Verification items for this drawing (mm, ordinates from the low corner). Round coordinates to 2 decimals unless told otherwise and drop trailing zeros. Loops run counter-clockwise (first coordinate to the right, second up) from the corner with the lowest first, then second, coordinate; pieces in that order, holes last. Notation, with made-up numbers: M -28,88 L -22,88 A29 cw -22,125 Z; hole C 21.5,54.5 d1. An arc over 180 degrees is marked long. Answer in a Markdown table with one row per item. Add a question column.
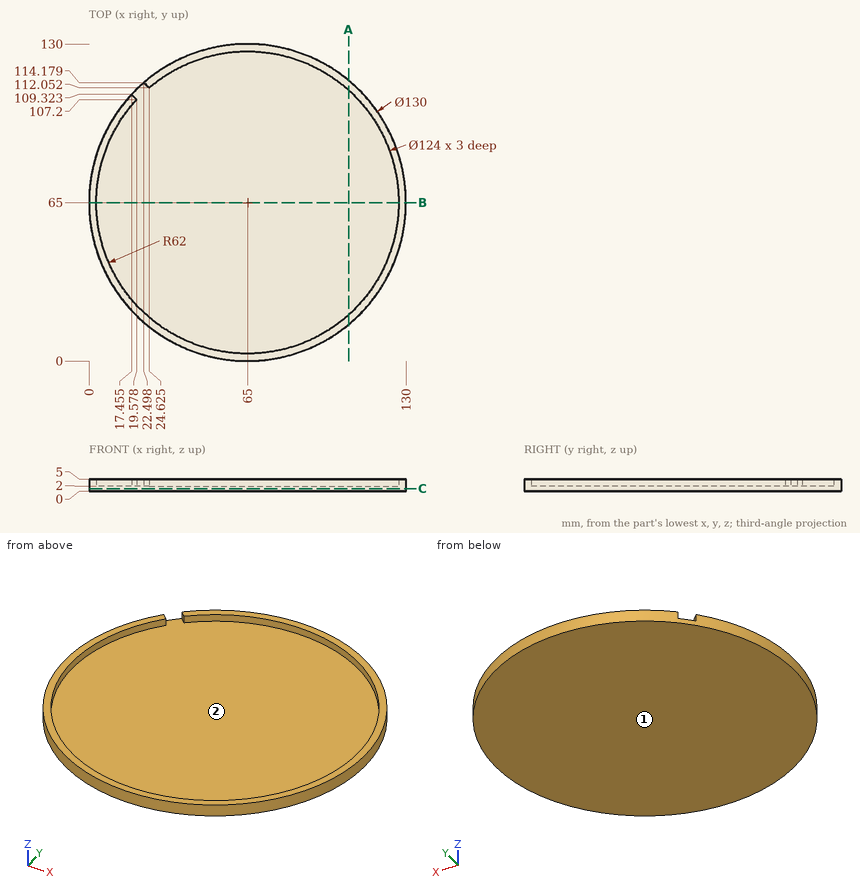
1) Cross-section at A-A, the plane x = 106.5. Record the boundary of the cut face in (y, z), plus the area to 3 significant figures.
2) Draft check along X on the marked faces 1 and 2. Enter one of: +X half, -X half, draft (parallel to the pull), parting line (faces both ways), or undercut.
3) Go/stop test with flat-tipped pins: pin 1 (1 mm diameter, centred on x = 41.5, z = 2, fed in from -Y) (1 decimal); pin 2 (1.5 mm diameter, centred on x = 25, z = 2, fed in from -Y); pin 3 (10 mm diameter, centred on x = 113.5, y = 84.5, fed in from +Z). Record where each tip stops, or that it passes through.
4) Thickness scan on L1, parallel to Y at x = 65, z = 3.2; L2, parallel to Z at x = 27.5, y = 65. Record the ranges inside material, lowest first. Write a range as [from, to].
5) Cross-section at B-B, the plane y = 65. Record the boundary of the cut face in (x, z), plus the area to 3 significant figures.
6) Cross-section at C-C, the plane z = 1. Record the boundary of the cut face in (x, y).
Worked answers:
| question | item | result |
|---|---|---|
| 1 | outline | M 14.97,0 L 115.03,0 L 115.03,5 L 111.06,5 L 111.06,2 L 18.94,2 L 18.94,5 L 14.97,5 Z |
| 1 | area | 224 mm2 |
| 2 | face 1 | draft |
| 2 | face 2 | undercut |
| 3 | pin 1 | stops at y = 4.2 |
| 3 | pin 2 | stops at y = 13.19 |
| 3 | pin 3 | stops at z = 2 |
| 4 | L1 | y = [0, 3], [127, 130] |
| 4 | L2 | z = [0, 2] |
| 5 | outline | M 0,0 L 130,0 L 130,5 L 127,5 L 127,2 L 3,2 L 3,5 L 0,5 Z |
| 5 | area | 278 mm2 |
| 6 | outline | C 65,65 d130 |
